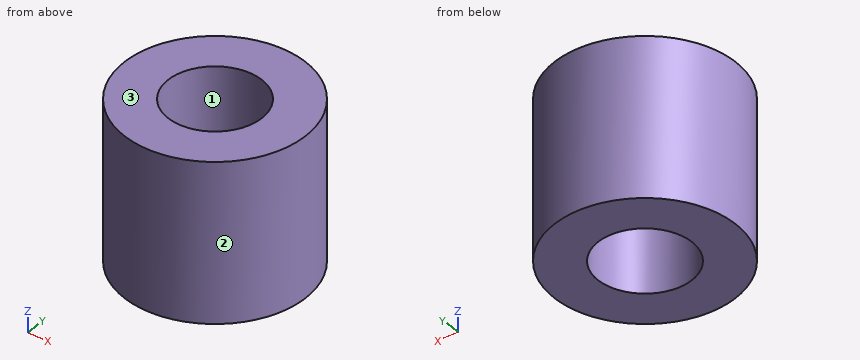
```python
from build123d import *

# Parameters (mm, degrees)
F0_R     = 54.840067
F1_DEPTH = 48.006
F2_R     = 26.964894
F3_DEPTH = 75.946
F4_R     = 28.396235
F5_DEPTH = 97.028


with BuildPart() as f1:
    # F0 (on Top) → F1 (new body, symmetric)
    with BuildSketch(Plane.XY):
        Circle(F0_R)
    extrude(amount=F1_DEPTH, both=True)

    # F2 (on face) → F3 (join)
    with BuildSketch(Plane.XY.offset(48.006)):
        Circle(F2_R)
    extrude(amount=-F3_DEPTH)

    # F4 (on face) → F5 (cut)
    with BuildSketch(Plane.XY.offset(48.006)):
        Circle(F4_R)
    extrude(amount=-F5_DEPTH, mode=Mode.SUBTRACT)


solid = f1.part
```
Read the model definition and answer for the solid it produces. Units are mm, in the model's axes. Face numbers are marked on the shaded views. Give positions to 0.01 mm unless a question says otherwise; leave off trailing zeros. Loops run counter-clockwise (first coordinate to the right, second up) from the corner with the lowest first, then second, coordinate; pieces in that order, holes last.
Item 1: Each of these flat-tipped pins is pushed along its axis until it touches: pin 1 Ø3 at (y, z) = (36, 33.5) entering from -X; pin 2 Ø3 at (x, z) = (7, 23) entering from -Y; pin 3 Ø8 at (y, z) = (-13, 23.5) entering from +X. Where does it stop, or does it pass through?
Item 2: The part is cut by section C-C (z = -37). Write down the section's boundary in (x, y).
Item 3: The part is cut by section A-A (x = 0). Write down the section's boundary in (y, z), and give its area (3 significant figures).
Item 4: The part is cut by section D-D (y = -42). Write down the section's boundary in (x, z).
Item 5: Find the intervals of material crossed by line 1 along Y through (x, z) = (0, -25); line 2 along X through (y, z) = (15, 13.5); line 3 along X through (y, z) = (-9.5, 36.5), in increasing order.
Item 6: The mould has two halves that part along Y. Classify the marked faces 1, 2 and 3: released by +Y, released by -Y, zero draft, split by the parting line, or undercut.
Taken from the geometry:
1. pin 1: stops at x = -42.63
1. pin 2: stops at y = -54.56
1. pin 3: stops at x = 54.1
2. outline: circle Ø109.68 at (0, 0); hole circle Ø56.79 at (0, 0)
3. outline: (-54.84, -48.01) - (-28.4, -48.01) - (-28.4, 48.01) - (-54.84, 48.01) - close; (28.4, -48.01) - (54.84, -48.01) - (54.84, 48.01) - (28.4, 48.01) - close
3. area: 5,080 mm2
4. outline: (-35.26, -48.01) - (35.26, -48.01) - (35.26, 48.01) - (-35.26, 48.01) - close
5. line 1: y = -54.84 to -28.4, 28.4 to 54.84
5. line 2: x = -52.75 to -24.11, 24.11 to 52.75
5. line 3: x = -54.01 to -26.76, 26.76 to 54.01
6. face 1: undercut
6. face 2: split by the parting line
6. face 3: zero draft
